For this review, take the finished solid that the model builds, in its own axes (mm). Face numbers are marked on the shaded views. A direction names the side the tool comes from. Round coordinates to 2 decimals unless told otherwise and drop trailing zeros. Order: outer loops, then holes, each group sorted by start corner. A loop starts at its lowest first (then second) coordinate and runs counter-clockwise, first axis right, second up. Notation, with made-up numbers: (56, 74.25) - (103, 74.25) arc R9 ccw to (103, 83.25) - close; hole circle Ø9 at (54, -7.5). An arc over 180 degrees is marked (long way). One line per question, with ' | ' between items.
```python
from build123d import *

# Parameters (mm, degrees)
BOSS_EXTRUDE1_DEPTH = 50


with BuildPart() as part:
    # Sketch1 → Boss-Extrude1 (new body)
    with BuildSketch(Plane.XY):
        with BuildLine():
            Line((0, 0), (-200, 0))
            ThreePointArc((-200, 0), (-300, 38.196601125), (-400, 0))
            Line((-400, 0), (-600, 0))
            Line((-600, 0), (-600, 50))
            Line((-600, 50), (-700, 50))
            Line((-700, 50), (-700, 55))
            Line((-700, 55), (-595, 55))
            Line((-595, 55), (-595, 5))
            Line((-595, 5), (-401.891933004, 5))
            ThreePointArc((-401.891933004, 5), (-300, 43.196601125), (-198.108066996, 5))
            Line((-198.108066996, 5), (0, 5))
            Line((0, 5), (0, 0))
        make_face()
    extrude(amount=BOSS_EXTRUDE1_DEPTH)


solid = part.part
```
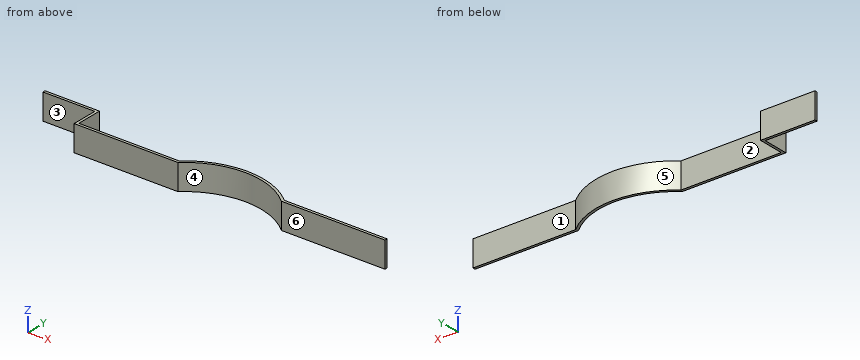
(1) Insertion check: pin 1 (5 mm diameter, centred on y = 6, z = 15.5, fed in from -X); pin 2 (8 mm diameter, centred on y = 9.5, z = 22, fed in from +X); pin 3 (15 mm diameter, centred on x = -123.5, z = 22, fed in from +Y). Each pin has a flat end and moves straight along its axis. Give the tip position at first contact, or say it passes through.
Output values:
pin 1: x = -600 | pin 2: x = -198.68 | pin 3: y = 5
(2) For probe 1 along X at (y, z) = (15, 25); probe 2 along Y at (x, z) = (-653, 13); probe 3 along X at (y, z) = (23.5, 24), list the stretches that pass through material, from the lowest coordinate up. Write a range as [from, to].
Output values:
probe 1: [-600, -595], [-389.14, -380.13], [-219.87, -210.86] | probe 2: [50, 55] | probe 3: [-600, -595], [-375.62, -364.75], [-235.25, -224.38]
(3) We need section D-D on x = -305. State the section outline as (y, z) points.
Output values:
outline: (38.11, 0) - (43.12, 0) - (43.12, 50) - (38.11, 50) - close
(4) We need section A-A on y = 12. State the section outline as (x, z) points, plus the area to 3 significant figures.
Output values:
outline: (-600, 0) - (-595, 0) - (-595, 50) - (-600, 50) - close; (-393.26, 0) - (-384.69, 0) - (-384.69, 50) - (-393.26, 50) - close; (-215.31, 0) - (-206.74, 0) - (-206.74, 50) - (-215.31, 50) - close | area: 1,110 mm^2
(5) Mouldability with a two-part tool opening along X and no side actions: class the marked faces 5 and 6 as released by +X, released by -X, zero draft, split by the parting line, or undercut.
Output values:
face 5: undercut | face 6: zero draft
(6) We need section B-B on z = 23. State the section outline as (x, y) points, plus the area to 3 significant figures.
Output values:
outline: (-700, 50) - (-600, 50) - (-600, 0) - (-400, 0) arc R150 cw to (-200, 0) - (0, 0) - (0, 5) - (-198.11, 5) arc R155 ccw to (-401.89, 5) - (-595, 5) - (-595, 55) - (-700, 55) - close | area: 3,840 mm^2
(7) For the marked faces 1, 2, 3 and 4, list the 3-axis set-ups (+Z, -Z, +X, -X, +Y, -Y) from which the entire face can be reached by the end or side of a thin tool; tool diameter is ignored.
Output values:
face 1: +Z, -Z, +X, +Y | face 2: +Z, -Z, +Y | face 3: +Z, -Z, -X, -Y | face 4: +Z, -Z, -Y
(8) We need section C-C on x = -561.5. State the section outline as (y, z) points.
Output values:
outline: (0, 0) - (5, 0) - (5, 50) - (0, 50) - close
